Check sheet for the modelled part. Datum: model origin and axes. Units: mm. Face numbers are marked on the shaded views. A direction names the side the tool comes from. Round coordinates to 2 decimals unless told otherwise and drop trailing zeros. Write each loop counter-clockwise with the first axis right and the second up, starting at its lowest first coordinate (ties: lowest second). Pieces come first, ordered by that corner, then holes. Notation, with made-up numbers: (67, -37.5) -> (73, -37.5) arc R9 cw to (73, -28.5) -> close; hole circle Ø2 at (88, 7.5). An arc over 180 degrees is marked (long way). Use one line per item in the form item = value. Start each with the question number.
```python
from build123d import *

# Parameters (mm, degrees)
SKETCH1_R                   = 12.7
BOSS_EXTRUDE1_DEPTH         = 12.7
SKETCH2_R                   = 15.24
CUT_EXTRUDE1_DEPTH          = 9.525
F_1_4_0_25_DIAMETER_HOLE1_D = 6.35


with BuildPart() as part:
    # Sketch1 → Boss-Extrude1 (new body)
    with BuildSketch(Plane.XY):
        Polygon((38.1, 0), (-38.1, 0), (-38.1, 6.35), (-19.05, 6.35), (-19.05, 44.45), (19.05, 44.45), (19.05, 6.35), (38.1, 6.35), align=None)
        with Locations((0, 25.4)):
            Circle(SKETCH1_R, mode=Mode.SUBTRACT)
    extrude(amount=BOSS_EXTRUDE1_DEPTH)

    # Sketch2 → Cut-Extrude1 (cut)
    with BuildSketch(Plane.XY.offset(12.7)):
        with Locations((0, 25.4)):
            Circle(SKETCH2_R)
    extrude(amount=-CUT_EXTRUDE1_DEPTH, mode=Mode.SUBTRACT)

    # 1/4 (0.25) Diameter Hole1 (through all)
    with Locations(Plane(origin=(-28.575, 6.35, 6.35), x_dir=(1, 0, 0), z_dir=(0, 1, 0))):
        with Locations((0, 0), (57.15, 0)):
            Hole(F_1_4_0_25_DIAMETER_HOLE1_D / 2)


solid = part.part
```
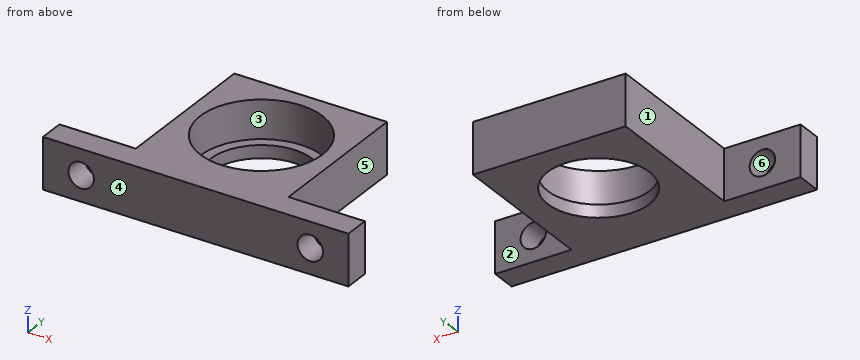
1. Mould release check, pull along X, two halves, no side actions. Record for the marked faces 4, 5 and 6: +X half, -X half, draft (parallel to the pull), parting line (faces both ways), or undercut.
2. Scan lines: probe 1 along Y at (x, z) = (0, 6); probe 2 along Y at (x, z) = (0, 0.95); probe 3 along Y at (x, z) = (-22, 2.75). Record each from-to range of solid material in increasing order.
3. Tool access check on the marked faces 1, 2 and 3. Record the directions out of +Z, -Z, +X, -X, +Y, -Y that give a thin tool (end or side, any length) a straight path to the whole face; none if there is none.
4. Sectioned sample at C-C (x = -6). Enter the section's corners in (y, z) (3 decimals).
5. Sectioned sample at D-D (y = 9). Enter the section's corners in (x, z), and give its area (3 significant figures).
6. Sectioned sample at B-B (y = 25.4). Enter the section's corners in (x, z) (3 decimals), and give its area (3 significant figures).
7. Depth check by flat-ended pin: pin 1 (4 mm diameter, centred on y = 17, z = 4.5, fed in from -X); pin 2 (3 mm diameter, centred on x = 21.5, z = 8.5, fed in from -Y); pin 3 (5 mm diameter, centred on y = 26, z = 11, fed in from +X); pin 4 (4 mm diameter, centred on x = -29.5, z = 9, fed in from +Y). Enter the tip coordinate at first touch or a pass-through.
8. Sectioned sample at A-A (z = 6.35). Enter the section's corners in (x, y), and give its area (3 significant figures).
Returned:
q1.face_4 = draft
q1.face_5 = +X half
q1.face_6 = undercut
q2.probe_1 = 0 to 10.16, 40.64 to 44.45
q2.probe_2 = 0 to 12.7, 38.1 to 44.45
q2.probe_3 = 0 to 6.35
q3.face_1 = +Z, -Z, -X, +Y
q3.face_2 = +Z, -Z, +X, +Y
q3.face_3 = +Z
q4.outline = (0, 0) -> (14.207, 0) -> (14.207, 3.175) -> (11.391, 3.175) -> (11.391, 12.7) -> (0, 12.7) -> close; (36.593, 0) -> (44.45, 0) -> (44.45, 12.7) -> (39.409, 12.7) -> (39.409, 3.175) -> (36.593, 3.175) -> close
q5.outline = (-19.05, 0) -> (19.05, 0) -> (19.05, 12.7) -> (-19.05, 12.7) -> close
q5.area = 484 mm^2
q6.outline = (-19.05, 0) -> (-12.7, 0) -> (-12.7, 3.175) -> (-15.24, 3.175) -> (-15.24, 12.7) -> (-19.05, 12.7) -> close; (12.7, 0) -> (19.05, 0) -> (19.05, 12.7) -> (15.24, 12.7) -> (15.24, 3.175) -> (12.7, 3.175) -> close
q6.area = 113 mm^2
q7.pin_1 = -19.05
q7.pin_2 = 0
q7.pin_3 = 19.05
q7.pin_4 = 6.35
q8.outline = (-38.1, 0) -> (-31.75, 0) -> (-31.75, 6.35) -> (-38.1, 6.35) -> close; (-25.4, 0) -> (25.4, 0) -> (25.4, 6.35) -> (19.05, 6.35) -> (19.05, 44.45) -> (-19.05, 44.45) -> (-19.05, 6.35) -> (-25.4, 6.35) -> close; (31.75, 0) -> (38.1, 0) -> (38.1, 6.35) -> (31.75, 6.35) -> close; hole circle Ø30.48 at (0, 25.4)
q8.area = 1,130 mm^2
